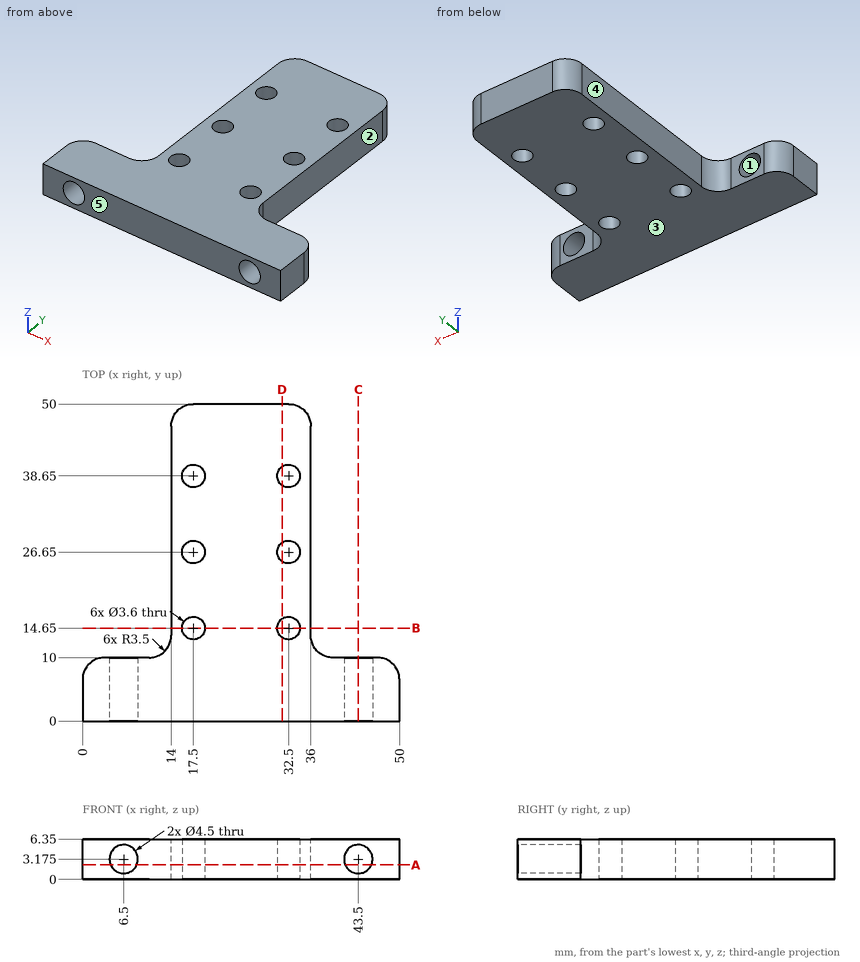
Design review of the part shown in the three views and the two pictorial views. Dimensions are in mm from the part's minimum x, y and z. A direction names the side the tool comes from. Round coordinates to 2 decimals unless told otherwise and drop trailing zeros. Loops run counter-clockwise (first coordinate to the right, second up) from the corner with the lowest first, then second, coordinate; pieces in that order, holes last. Notation, with made-up numbers: (-1, 77.5) -> (5, 77.5) arc R25 ccw to (5, 95.5) -> close; hole circle Ø6 at (73.5, -9.5). An arc over 180 degrees is marked (long way). Use one line per item in the form item = value. Start each with the question number.
Q1. We need section B-B on y = 14.65. Give the boundary of the cut face in (x, z).
Q2. We need section C-C on x = 43.5. Give the boundary of the cut face in (y, z) (3 decimals).
Q3. We need section A-A on z = 2.25. State how many separate pieces and enclosed holes the cut face has, then the cut area to 3 significant figures.
Q4. Machinability: for the marked faces 4 and 5, which of the approach directions +Z, -Z, +X, -X, +Y, -Y give a long, thin tool a straight path to every point of the face, cutting with its end or side? Answer none if there is none.
Q5. Draft analysis for pull direction Z (two halves, no side actions). For the marked faces 1, 2 and 3, state which applies: +Z half, -Z half, draft (parallel to the pull), parting line (faces both ways), or undercut.
Q6. We need section D-D on x = 31.5. Give the boundary of the cut face in (y, z).
Q7. Wall thickness on line 1 along Y through (x, z) = (17.5, 5); line 2 along X through (y, z) = (14, 5.5); line 3 along X through (y, z) = (40, 3.5): over which ranges is each line inside the solid? List them lowest first. Write a range as [from, to].
Q8. For pin 1 Ø2.5 at (x, z) = (6.5, 3.175) entering from +Y; pin 2 Ø1.5 at (x, z) = (42.5, 1.5) entering from +Y; pin 3 Ø1.9 at (y, z) = (24.5, 2.5) entering from +X; pin 4 Ø2 at (y, z) = (22, 4.5) entering from -X, all flat-tipped, find the tip position at first contact; note any pin that passes through.
Calculated:
q1.outline = (14, 0) -> (15.7, 0) -> (15.7, 6.35) -> (14, 6.35) -> close; (19.3, 0) -> (30.7, 0) -> (30.7, 6.35) -> (19.3, 6.35) -> close; (34.3, 0) -> (36, 0) -> (36, 6.35) -> (34.3, 6.35) -> close
q2.outline = (0, 0) -> (10, 0) -> (10, 0.925) -> (0, 0.925) -> close; (0, 5.425) -> (10, 5.425) -> (10, 6.35) -> (0, 6.35) -> close
q3.separate_pieces = 3
q3.enclosed_holes = 6
q3.area = 1,230 mm²
q4.face_4 = +Z, -Z, -X, +Y
q4.face_5 = +Z, -Z, +X, -X, -Y
q5.face_1 = undercut
q5.face_2 = draft
q5.face_3 = -Z half
q6.outline = (0, 0) -> (13.15, 0) -> (13.15, 6.35) -> (0, 6.35) -> close; (16.15, 0) -> (25.15, 0) -> (25.15, 6.35) -> (16.15, 6.35) -> close; (28.15, 0) -> (37.15, 0) -> (37.15, 6.35) -> (28.15, 6.35) -> close; (40.15, 0) -> (50, 0) -> (50, 6.35) -> (40.15, 6.35) -> close
q7.line_1 = [0, 12.85], [16.45, 24.85], [28.45, 36.85], [40.45, 50]
q7.line_2 = [14, 15.82], [19.18, 30.82], [34.18, 36]
q7.line_3 = [14, 16.31], [18.69, 31.31], [33.69, 36]
q8.pin_1 = through
q8.pin_2 = 10
q8.pin_3 = 36
q8.pin_4 = 14
